Input: dimensioned drawing with shaded views. Units: mm. Origin: part minimum x, y, z. Give positions to 0.01 mm unless a question says otherwise; leave off trailing zeros. Order: outer loops, then holes, each group sorted by start corner. A loop starts at its lowest first (then second) coordinate and runs counter-clockwise, first axis right, second up.
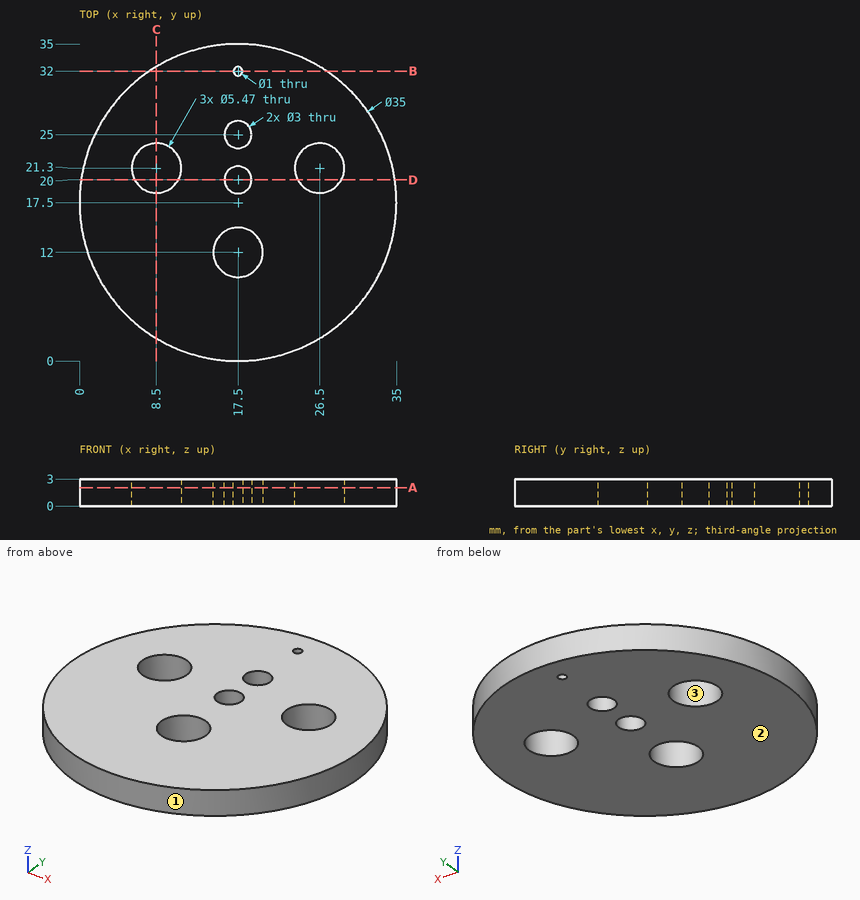
1) Pull-direction query (Y, two-part tool) for the marked faces 1, 2 and 3; classes: pulls with the +Y half, pulls with the -Y half, needs draft (parallel to the pull), parting line crosses it, or undercut.
2) First-contact query: P1, Ø1, axis at x = 24.5, z = 0.5, coming from the -Y side. Flat tip, straight axial feed; report the tip coordinate or a pass-through.
3) Cut plane C-C (x = 8.5). Return the cut outline in (y, z) (3 decimals).
4) Cut plane B-B (y = 32). Return the cut outline in (x, z).
5) Cut plane A-A (z = 2.05). Return the cut outline in (x, y) (3 decimals), then the cut area to 3 significant figures.
6) Cut plane D-D (y = 20). Return the cut outline in (x, z).
7) Line query: probe 1 along Y at (x, z) = (17.5, 2.3) (3 decimals); probe 2 along X at (y, z) = (32, 0.75); probe 3 along Y at (x, z) = (8.5, 1.85) (3 decimals). Output: solid intervals per line, ascending.
Geometry says:
1. face 1: parting line crosses it
1. face 2: needs draft
1. face 3: undercut
2. P1: stops at y = 1.25
3. outline: (2.492, 0) - (18.565, 0) - (18.565, 3) - (2.492, 3) - close; (24.035, 0) - (32.508, 0) - (32.508, 3) - (24.035, 3) - close
4. outline: (7.7, 0) - (17, 0) - (17, 3) - (7.7, 3) - close; (18, 0) - (27.3, 0) - (27.3, 3) - (18, 3) - close
5. outline: circle Ø35 at (17.5, 17.5); hole circle Ø5.47 at (8.5, 21.3); hole circle Ø5.47 at (17.5, 12); hole circle Ø3 at (17.5, 20); hole circle Ø3 at (17.5, 25); hole circle Ø1 at (17.5, 32); hole circle Ø5.47 at (26.5, 21.3)
5. area: 877 mm2
6. outline: (0.18, 0) - (6.09, 0) - (6.09, 3) - (0.18, 3) - close; (10.91, 0) - (16, 0) - (16, 3) - (10.91, 3) - close; (19, 0) - (24.09, 0) - (24.09, 3) - (19, 3) - close; (28.91, 0) - (34.82, 0) - (34.82, 3) - (28.91, 3) - close
7. probe 1: y = 0 to 9.265, 14.735 to 18.5, 21.5 to 23.5, 26.5 to 31.5, 32.5 to 35
7. probe 2: x = 7.7 to 17, 18 to 27.3
7. probe 3: y = 2.492 to 18.565, 24.035 to 32.508
